Autodesk Inventor part; units mm, degrees
ref_plane "YZ Plane" through (0, 0, 0) normal (1, 0, 0) x (0, 1, 0)
ref_plane "XZ Plane" through (0, 0, 0) normal (0, 1, 0) x (-1, 0, 0)
ref_plane "XY Plane" through (0, 0, 0) normal (0, 0, 1) x (1, 0, 0)
sketch "Sketch1" plane through (0, 0, 0) normal (0, 1, 0) x (-1, 0, 0)
  line L0 (0, 0) -> (-32, 0)
  line L1 (-32, 0) -> (-32, -30)
  line L2 (-32, -30) -> (0, -30)
  line L3 (0, -30) -> (0, 0)
  dimension "d0" = 30
  dimension "d1" = 32
extrude "Extrusion1" add sketch "Sketch1" along normal blind 3
sketch "Sketch2" plane through (0, 3, 0) normal (0, 1, 0) x (1, 0, 0)
  line L0 (0, 0) -> (32, 0)
  line L1 (32, 0) -> (32, 30)
  line L2 (32, 30) -> (0, 30)
  line L3 (0, 30) -> (0, 0)
  line L4 (9.25, 20.5) -> (22.75, 20.5)
  line L5 (22.75, 20.5) -> (22.75, 9.5)
  line L6 (22.75, 9.5) -> (9.25, 9.5)
  line L7 (9.25, 9.5) -> (9.25, 20.5)
  point P0 (9.25, 15)
  point P1 (0, 15)
  point P2 (16, 9.5)
  point P3 (16, 0)
  dimension "d4" = 11
  dimension "d5" = 13.5
extrude "Extrusion2" add sketch "Sketch2" along normal blind 5.5
sketch "Sketch3" plane through (0, 8.5, 0) normal (0, 1, 0) x (1, 0, 0)
  line L0 (22.75, 20.5) -> (22.75, 9.5)
  line L1 (32, 0) -> (32, 30)
  line L2 (22.75, 17.5) -> (32, 17.5)
  line L3 (32, 17.5) -> (32, 12.5)
  line L4 (32, 12.5) -> (22.75, 12.5)
  line L5 (22.75, 12.5) -> (22.75, 17.5)
  point P0 (22.75, 15)
  point P1 (22.75, 15)
  dimension "d8" = 5
extrude "Extrusion3" cut sketch "Sketch3" against normal up to surface (5.5 mm away)
sketch "Sketch4" plane through (0, 8.5, 0) normal (0, 1, 0) x (1, 0, 0)
  line L0 (32, 30) -> (0, 30)
  line L1 (0, 30) -> (0, 0)
  line L2 (6, 24) -> (26, 24) construction
  line L3 (26, 24) -> (26, 6) construction
  line L4 (26, 6) -> (6, 6) construction
  line L5 (6, 6) -> (6, 24) construction
  circle A0 centre (6, 24) radius 2
  circle A1 centre (6, 6) radius 2
  circle A2 centre (26, 6) radius 2
  circle A3 centre (26, 24) radius 2
  point P0 (6, 15)
  point P1 (0, 15)
  point P2 (16, 24)
  point P3 (16, 30)
  dimension "d11" = 4
  dimension "d18" = 18
  dimension "d19" = 20
extrude "Extrusion4" cut sketch "Sketch4" against normal through all
fillet "Fillet1" radius 6 4 edges at (0, 4.25, -30) (0, 4.25, 0) (32, 4.25, 0) (32, 4.25, -30)
sketch "Sketch5" plane through (0, 0, 0) normal (0, -1, 0) x (1, 0, 0)
  circle A0 centre (26, -6) radius 2
  circle A1 centre (6, -24) radius 2
  circle A2 centre (6, -6) radius 2
  circle A3 centre (26, -24) radius 2
  line L0 (3.9793, -9.5) -> (1.9585, -6)
  line L1 (1.9585, -6) -> (3.9793, -2.5)
  line L2 (3.9793, -2.5) -> (8.0207, -2.5)
  line L3 (8.0207, -2.5) -> (10.0415, -6)
  line L4 (10.0415, -6) -> (8.0207, -9.5)
  line L5 (8.0207, -9.5) -> (3.9793, -9.5)
  line L6 (8.0207, -20.5) -> (10.0415, -24)
  line L7 (10.0415, -24) -> (8.0207, -27.5)
  line L8 (8.0207, -27.5) -> (3.9793, -27.5)
  line L9 (3.9793, -27.5) -> (1.9585, -24)
  line L10 (1.9585, -24) -> (3.9793, -20.5)
  line L11 (3.9793, -20.5) -> (8.0207, -20.5)
  line L12 (21.9585, -24) -> (23.9793, -20.5)
  line L13 (23.9793, -20.5) -> (28.0207, -20.5)
  line L14 (28.0207, -20.5) -> (30.0415, -24)
  line L15 (30.0415, -24) -> (28.0207, -27.5)
  line L16 (28.0207, -27.5) -> (23.9793, -27.5)
  line L17 (23.9793, -27.5) -> (21.9585, -24)
  line L18 (21.9585, -6) -> (23.9793, -2.5)
  line L19 (23.9793, -2.5) -> (28.0207, -2.5)
  line L20 (28.0207, -2.5) -> (30.0415, -6)
  line L21 (30.0415, -6) -> (28.0207, -9.5)
  line L22 (28.0207, -9.5) -> (23.9793, -9.5)
  line L23 (23.9793, -9.5) -> (21.9585, -6)
  point P0 (0, 0)
  point P1 (6, -27.5)
  dimension "d21" = 7
extrude "Extrusion5" cut sketch "Sketch5" against normal blind 6
properties part number "bottom"
Work out the finished part from the listing and answer in its coordinate system (mm). A direction names the side the tool comes from. Give positions to 0.01 mm unless a question says otherwise; leave off trailing zeros. Loops run counter-clockwise (first coordinate to the right, second up) from the corner with the lowest first, then second, coordinate; pieces in that order, holes last. Notation, with made-up numbers: (66, 43) -> (96, 43) arc R18 ccw to (96, 68) -> close; hole circle Ø2 at (-24.75, 87). An arc over 180 degrees is marked (long way). Use a Markdown table: item, result. Add a question column.
1. Section B-B on z = -10.5 is taken. Determine the outline of the cut face in (x, y), and give its area (3 significant figures).
2. Section D-D on x = 3.5 is taken. Determine the outline of the cut face in (y, z).
3. Section A-A on y = 6.5 is taken. Determine the outline of the cut face in (x, z), and give its area (3 significant figures).
4. Section C-C on x = 7 is taken. Determine the outline of the cut face in (y, z), and give its area (3 significant figures).
5. A flat-ended cylindrical pin translates along its axis: pin 1 Ø1 at (x, z) = (20, -16.5) entering from +Y. Find the tip coordinate at first contact, or state that the pin passes through.
6. Find the intervals of material crossed by probe 1 along Z at (x, y) = (6, 7.05); probe 2 along X at (y, z) = (7, -24); probe 3 along Z at (x, y) = (26, 7.1), in increasing order.
7. For faces 1 (the flat face through (32, 2, -15)), 2 (the flat face through (9.045, 2.958, -25.726)), 3 (the flat face through (27, 6, -17.5)), determine the directions among +Z, -Z, +X, -X, +Y, -Y from which every point of the face is accessible in a straight line to the end or side of a thin tool.
Results below:
| question | item | result |
|---|---|---|
| 1 | outline | (0, 0) -> (32, 0) -> (32, 8.5) -> (22.75, 8.5) -> (22.75, 3) -> (9.25, 3) -> (9.25, 8.5) -> (0, 8.5) -> close |
| 1 | area | 198 mm^2 |
| 2 | outline | (0, -29.45) -> (8.5, -29.45) -> (8.5, -0.55) -> (0, -0.55) -> (0, -3.33) -> (6, -3.33) -> (6, -8.67) -> (0, -8.67) -> (0, -21.33) -> (6, -21.33) -> (6, -26.67) -> (0, -26.67) -> close |
| 3 | outline | (0, -24) arc R6 ccw to (6, -30) -> (26, -30) arc R6 ccw to (32, -24) -> (32, -17.5) -> (22.75, -17.5) -> (22.75, -20.5) -> (9.25, -20.5) -> (9.25, -9.5) -> (22.75, -9.5) -> (22.75, -12.5) -> (32, -12.5) -> (32, -6) arc R6 ccw to (26, 0) -> (6, 0) arc R6 ccw to (0, -6) -> close; hole circle Ø4 at (6, -24); hole circle Ø4 at (6, -6); hole circle Ø4 at (26, -24); hole circle Ø4 at (26, -6) |
| 3 | area | 684 mm^2 |
| 4 | outline | (0, -30) -> (8.5, -30) -> (8.5, -25.73) -> (6, -25.73) -> (6, -27.5) -> (0, -27.5) -> close; (0, -20.5) -> (6, -20.5) -> (6, -22.27) -> (8.5, -22.27) -> (8.5, -7.73) -> (6, -7.73) -> (6, -9.5) -> (0, -9.5) -> close; (0, -2.5) -> (6, -2.5) -> (6, -4.27) -> (8.5, -4.27) -> (8.5, 0) -> (0, 0) -> close |
| 4 | area | 154 mm^2 |
| 5 | pin 1 | stops at y = 3 |
| 6 | probe 1 | z = -30 to -26, -22 to -8, -4 to 0 |
| 6 | probe 2 | x = 0 to 4, 8 to 24, 28 to 32 |
| 6 | probe 3 | z = -30 to -26, -22 to -17.5, -12.5 to -8, -4 to 0 |
| 7 | face 1 | +Z, -Z, +X, +Y, -Y |
| 7 | face 2 | -Y |
| 7 | face 3 | +X, +Y |
